```python
from build123d import *

# Parameters (mm, degrees)
SKETCH1_R           = 2.4892
BOSS_EXTRUDE1_DEPTH = 3.175


with BuildPart() as part:
    # Sketch1 → Boss-Extrude1 (new body)
    with BuildSketch(Plane(origin=(0, 0, 0), x_dir=(1, 0, 0), z_dir=(0, 1, 0))):
        Polygon((38.1, 0), (-38.1, 0), (-38.1, 25.4), (-12.7, 25.4), (-12.7, 76.2), (12.7, 76.2), (12.7, 25.4), (38.1, 25.4), align=None)
        with Locations((0, 63.5)):
            Circle(SKETCH1_R, mode=Mode.SUBTRACT)
        with Locations((0, 38.1)):
            Circle(SKETCH1_R, mode=Mode.SUBTRACT)
        with Locations((-25.4, 12.7)):
            Circle(SKETCH1_R, mode=Mode.SUBTRACT)
        with Locations((25.4, 12.7)):
            Circle(SKETCH1_R, mode=Mode.SUBTRACT)
        with Locations((0, 12.7)):
            Circle(SKETCH1_R, mode=Mode.SUBTRACT)
    extrude(amount=BOSS_EXTRUDE1_DEPTH)


solid = part.part
```
Part model, mm, in its own coordinate system. A direction names the side the tool comes from. Coordinates: 2 decimals unless noted, no trailing zeros. Order: outer loops, then holes, each group sorted by start corner. A loop starts at its lowest first (then second) coordinate and runs counter-clockwise, first axis right, second up. Notation, with made-up numbers: (-14, 65.25) - (-9, 65.25) arc R22 ccw to (-9, 102.25) - close; hole circle Ø5 at (82.25, 4.5). An arc over 180 degrees is marked (long way). Return JSON: item names as keys, results as strings. Group by question number.
Item 1: Cut at A-A (z = -38.1). List the corners of the cut face in (x, y) (3 decimals).
Item 2: Pull direction Z, two halves, no side cores. Call faces 4 (the face through (1, 3.175, -30)), 5 (the face through (-0.32, 1.57, -15.17)), 6 (the face through (1, 2, 0)): pulls with the +Z half, pulls with the -Z half, needs draft (parallel to the pull), parting line crosses it, or undercut.
Item 3: Pin check, flat tips, straight feed: pin 1 (1.6 mm diameter, centred on y = 1.5, z = -58, fed in from +X); pin 2 (1.6 mm diameter, centred on x = -22, y = 1.5, fed in from -Z); pin 3 (1 mm diameter, centred on y = 1.5, z = -44, fed in from -X). Stop position of each tip, or through.
Item 4: Cut at C-C (y = 2.6). List the corners of the cut face in (x, z).
Item 5: Cut at D-D (z = -12.7). List the corners of the cut face in (x, y) (3 decimals), plus the area to 3 significant figures.
Item 6: Drill centre lines: probe 1 along Z at (x, y) = (0, 2.05); probe 2 along X at (y, z) = (2.55, -12.7); probe 3 along X at (y, z) = (0.85, -38.1). Where is each one in solid material? Low to high. Write a range as from..to.
Item 7: Which spindle directions (+Z, -Z, +X, -X, +Y, -Y) get a long thin tool onto all of the face, cutting with end or side? Do faces 1 (the face through (12.7, 2, -51)), 2 (the face through (-38.1, 2, -13)), 3 (the face through (-12.7, 2, -50)). Say none if no direction does.
Item 8: Cut at B-B (x = 25.4). List the corners of the cut face in (y, z) (3 decimals), plus the area to 3 significant figures.
Check values:
{
 "1": {"outline": "(-12.7, 0) - (-2.489, 0) - (-2.489, 3.175) - (-12.7, 3.175) - close; (2.489, 0) - (12.7, 0) - (12.7, 3.175) - (2.489, 3.175) - close"},
 "2": {"face 4": "needs draft", "face 5": "undercut", "face 6": "pulls with the +Z half"},
 "3": {"pin 1": "stops at x = 12.7", "pin 2": "stops at z = -25.4", "pin 3": "stops at x = -12.7"},
 "4": {"outline": "(-38.1, -25.4) - (-12.7, -25.4) - (-12.7, -76.2) - (12.7, -76.2) - (12.7, -25.4) - (38.1, -25.4) - (38.1, 0) - (-38.1, 0) - close; hole circle Ø4.98 at (-25.4, -12.7); hole circle Ø4.98 at (0, -63.5); hole circle Ø4.98 at (0, -38.1); hole circle Ø4.98 at (0, -12.7); hole circle Ø4.98 at (25.4, -12.7)"},
 "5": {"outline": "(-38.1, 0) - (-27.889, 0) - (-27.889, 3.175) - (-38.1, 3.175) - close; (-22.911, 0) - (-2.489, 0) - (-2.489, 3.175) - (-22.911, 3.175) - close; (2.489, 0) - (22.911, 0) - (22.911, 3.175) - (2.489, 3.175) - close; (27.889, 0) - (38.1, 0) - (38.1, 3.175) - (27.889, 3.175) - close", "area": "195 mm2"},
 "6": {"probe 1": "z = -76.2..-65.99, -61.01..-40.59, -35.61..-15.19, -10.21..0", "probe 2": "x = -38.1..-27.89, -22.91..-2.49, 2.49..22.91, 27.89..38.1", "probe 3": "x = -12.7..-2.49, 2.49..12.7"},
 "7": {"face 1": "-Z, +X, +Y, -Y", "face 2": "+Z, -Z, -X, +Y, -Y", "face 3": "-Z, -X, +Y, -Y"},
 "8": {"outline": "(0, -25.4) - (3.175, -25.4) - (3.175, -15.189) - (0, -15.189) - close; (0, -10.211) - (3.175, -10.211) - (3.175, 0) - (0, 0) - close", "area": "64.8 mm2"}
}
